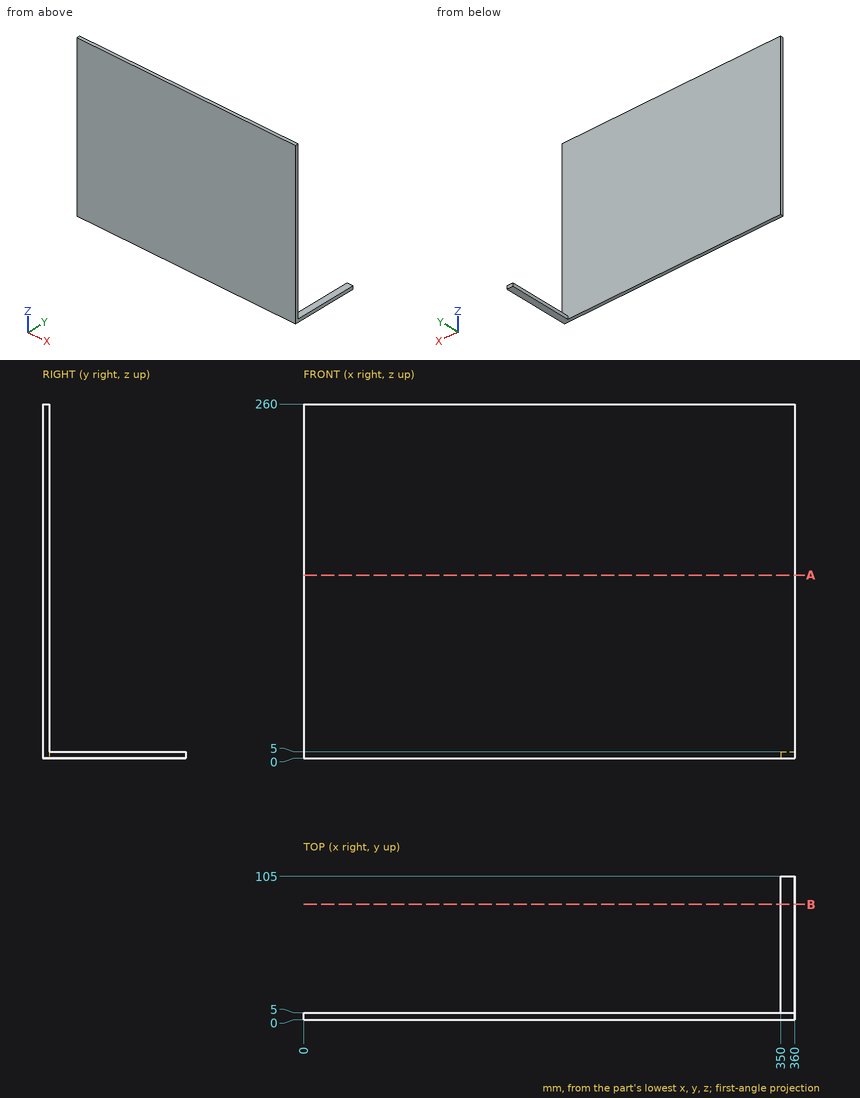
Here's the drawing with two shaded views (mm, measured from the low corner). I have some questions. Give positions to 0.01 mm unless a question says otherwise; leave off trailing zeros. Order: outer loops, then holes, each group sorted by start corner. A loop starts at its lowest first (then second) coordinate and runs counter-clockwise, first axis right, second up. Notation, with made-up numbers: (49, -22) -> (82, -22) arc R14 ccw to (82, 5) -> close; hole circle Ø3 at (3.5, 76). An arc over 180 degrees is marked (long way). Use a Markdown table: item, result. Add a question column.
Item 1: Imagine slicing it at B-B on y = 84.5. Please give me the cut outline in (x, z).
Item 2: I need wall thicknesses on line 1 (Y direction, x = 237, z = 23.5). Which ranges of the line are inside material? Lowest first, please.
Item 3: Imagine slicing it at A-A on z = 134.5. Please give me the cut outline in (x, y).
Item 4: Will these pins go through, and if not, where does the flat tip stop? pin 1 (8 mm diameter, centred on x = 357, y = 37.5, fed in from +Z); pin 2 (2 mm diameter, centred on x = 263.5, z = 211.5, fed in from +Y); pin 3 (4 mm diameter, centred on y = 46.5, z = 3.5, fed in from -X).
Data:
| question | item | result |
|---|---|---|
| 1 | outline | (350, 0) -> (360, 0) -> (360, 5) -> (350, 5) -> close |
| 2 | line 1 | y = 0 to 5 |
| 3 | outline | (0, 0) -> (360, 0) -> (360, 5) -> (0, 5) -> close |
| 4 | pin 1 | stops at z = 5 |
| 4 | pin 2 | stops at y = 5 |
| 4 | pin 3 | stops at x = 350 |
